Check sheet for the modelled part. Datum: model origin and axes. Units: mm. Face numbers are marked on the shaded views. A direction names the side the tool comes from. Coordinates: 2 decimals unless noted, no trailing zeros. Order: outer loops, then holes, each group sorted by start corner. A loop starts at its lowest first (then second) coordinate and runs counter-clockwise, first axis right, second up.
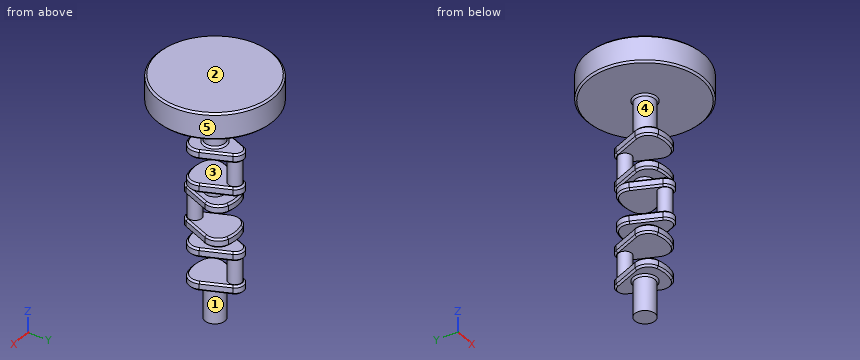
from build123d import *

# Parameters (mm, degrees)
SKETCH1_R             = 9.525
BOSS_EXTRUDE1_DEPTH   = 34.925
BOSS_EXTRUDE2_DEPTH   = 12.7
FILLET1_R             = 19.05
SKETCH3_R             = 14.2875
BOSS_EXTRUDE3_DEPTH   = 9.525
LPATTERN1_COUNT       = 3
LPATTERN1_PITCH       = 69.85
BODY_MOVE_COPY1_ANGLE = 180
LPATTERN2_COUNT       = 2
LPATTERN2_PITCH       = 69.85
SKETCH4_R             = 14.2875
BOSS_EXTRUDE4_DEPTH   = 57.15
BOSS_EXTRUDE5_START   = 50.8
SKETCH5_R             = 14.2875
BOSS_EXTRUDE5_DEPTH   = 50.8
SKETCH6_R             = 83.107085054
BOSS_EXTRUDE6_DEPTH   = 38.1
CHAMFER1_SIZE         = 2.54


with BuildPart() as part:
    # Sketch1 → Boss-Extrude1 (new body)
    with BuildSketch(Plane.XY):
        Circle(SKETCH1_R)
    extrude(amount=-BOSS_EXTRUDE1_DEPTH)

    # Sketch2 → Boss-Extrude2 (add)
    with BuildSketch(Plane(origin=(0, 0, -34.925), x_dir=(-1, 0, 0), z_dir=(0, 0, -1))):
        with BuildLine():
            Line((-11.733270063, 4.860079591), (-33.507418174, -47.707364088))
            ThreePointArc((-33.507418174, -47.707364088), (0, -60.325), (33.507418174, -47.707364088))
            Line((33.507418174, -47.707364088), (11.733270063, 4.860079591))
            ThreePointArc((11.733270063, 4.860079591), (0, 12.7), (-11.733270063, 4.860079591))
        make_face()
    extrude(amount=BOSS_EXTRUDE2_DEPTH)

    # Fillet1
    fillet1_edges = [part.edges().sort_by_distance(p)[0] for p in [
        (33.507418174, -47.707364088, -41.275),
        (-33.507418174, -47.707364088, -41.275),
    ]]
    fillet(fillet1_edges, radius=FILLET1_R)

    # Mirror2: part across plane


with BuildPart() as part_1:
    add(part.part)
    add(part.part.mirror(Plane.XY.offset(-17.4625)))


with BuildPart() as body_2:
    # Sketch3 → Boss-Extrude3 (new body)
    with BuildSketch(Plane(origin=(0, 0, -47.625), x_dir=(-1, 0, 0), z_dir=(0, 0, -1))):
        with Locations(Location((0, -28.486474017, 0), (0, 0, 180))):
            Circle(SKETCH3_R)
    boss_extrude3 = extrude(amount=BOSS_EXTRUDE3_DEPTH)


with BuildPart() as lpattern1_1:
    # LPattern1: pattern copy
    add(part_1.part.moved(Location(Vector(0, 0, -1) * (1 * LPATTERN1_PITCH))))


with BuildPart() as lpattern1_2:
    # LPattern1: pattern copy
    add(part_1.part.moved(Location(Vector(0, 0, -1) * (2 * LPATTERN1_PITCH))))

    # Sketch5 → Boss-Extrude5 (add)
    with BuildSketch(Plane(origin=(0, 0, -187.325), x_dir=(-1, 0, 0), z_dir=(0, 0, -1)).offset(BOSS_EXTRUDE5_START)):
        with Locations(Location((0, -28.486474017, 0), (0, 0, 180))):
            Circle(SKETCH5_R)
    extrude(amount=-BOSS_EXTRUDE5_DEPTH)


with BuildPart() as lpattern1_1_1:
    # Body-Move_Copy1: moved
    add(lpattern1_1.part.rotate(Axis((0, -28.486474017, 0), (0, 0, 1)), BODY_MOVE_COPY1_ANGLE))


with BuildPart() as lpattern2_1:
    # LPattern2: Boss-Extrude3 ×2
    with Locations(*[(0, 0, -i * LPATTERN2_PITCH) for i in range(1, LPATTERN2_COUNT)]):
        add(boss_extrude3)


with BuildPart() as part_2:
    add(part_1.part)

    # Sketch4 → Boss-Extrude4 (add)
    with BuildSketch(Plane.XY.offset(12.7)):
        with Locations((0, -28.486474017)):
            Circle(SKETCH4_R)
    extrude(amount=BOSS_EXTRUDE4_DEPTH)

    # Sketch6 → Boss-Extrude6 (add)
    with BuildSketch(Plane.XY.offset(69.85)):
        with Locations(Location((0, -28.486474017, 0), (0, 0, 180))):
            Circle(SKETCH6_R)
    extrude(amount=BOSS_EXTRUDE6_DEPTH)


with BuildPart() as body_2_1:
    add(body_2.part)

    # Combine1: union LPattern1_1, LPattern2_1, LPattern1_2, part
    add(lpattern1_1_1.part)
    add(lpattern2_1.part)
    add(lpattern1_2.part)
    add(part_2.part)

    # Chamfer1
    chamfer1_edges = [body_2_1.edges().sort_by_distance(p)[0] for p in [
        (0, -69.672948033, -104.775),
        (-19.470080331, -43.154715345, -104.775),
        (0, 3.352051967, -104.775),
        (19.470080331, -43.154715345, -104.775),
        (-19.470080331, -43.154715345, -117.475),
        (-26.88006293, -9.152399421, -117.475),
        (0, 3.352051967, -117.475),
        (26.88006293, -9.152399421, -117.475),
        (19.470080331, -43.154715345, -117.475),
        (0, -69.672948033, -117.475),
        (-26.88006293, -9.152399421, -104.775),
        (26.88006293, -9.152399421, -104.775),
        (0, -69.672948033, -57.15),
        (-19.470080331, -43.154715345, -57.15),
        (0, 3.352051967, -57.15),
        (19.470080331, -43.154715345, -57.15),
        (0, 3.352051967, -69.85),
        (19.470080331, -43.154715345, -69.85),
        (0, -69.672948033, -69.85),
        (-19.470080331, -43.154715345, -69.85),
        (-26.88006293, -9.152399421, -57.15),
        (-26.88006293, -9.152399421, -69.85),
        (26.88006293, -9.152399421, -57.15),
        (26.88006293, -9.152399421, -69.85),
        (0, 12.7, -174.625),
        (19.470080331, -13.818232688, -174.625),
        (0, -60.325, -174.625),
        (-19.470080331, -13.818232688, -174.625),
        (19.470080331, -13.818232688, -187.325),
        (26.88006293, -47.820548612, -187.325),
        (0, -60.325, -187.325),
        (-26.88006293, -47.820548612, -187.325),
        (-19.470080331, -13.818232688, -187.325),
        (0, 12.7, -187.325),
        (26.88006293, -47.820548612, -174.625),
        (-26.88006293, -47.820548612, -174.625),
        (0, 12.7, -127),
        (19.470080331, -13.818232688, -127),
        (0, -60.325, -127),
        (-19.470080331, -13.818232688, -127),
        (0, -60.325, -139.7),
        (-19.470080331, -13.818232688, -139.7),
        (0, 12.7, -139.7),
        (19.470080331, -13.818232688, -139.7),
        (26.88006293, -47.820548612, -127),
        (26.88006293, -47.820548612, -139.7),
        (-26.88006293, -47.820548612, -127),
        (-26.88006293, -47.820548612, -139.7),
        (-14.2875, -28.486474017, -187.325),
        (0, 12.7, -34.925),
        (19.470080331, -13.818232688, -34.925),
        (0, -60.325, -34.925),
        (-19.470080331, -13.818232688, -34.925),
        (19.470080331, -13.818232688, -47.625),
        (26.88006293, -47.820548612, -47.625),
        (0, -60.325, -47.625),
        (-26.88006293, -47.820548612, -47.625),
        (-19.470080331, -13.818232688, -47.625),
        (0, 12.7, -47.625),
        (26.88006293, -47.820548612, -34.925),
        (-26.88006293, -47.820548612, -34.925),
        (0, 12.7, 12.7),
        (19.470080331, -13.818232688, 12.7),
        (0, -60.325, 12.7),
        (-19.470080331, -13.818232688, 12.7),
        (0, -60.325, 0),
        (-19.470080331, -13.818232688, 0),
        (0, 12.7, 0),
        (19.470080331, -13.818232688, 0),
        (26.88006293, -47.820548612, 12.7),
        (26.88006293, -47.820548612, 0),
        (-26.88006293, -47.820548612, 12.7),
        (-26.88006293, -47.820548612, 0),
        (-14.2875, -28.486474017, 12.7),
        (83.107085054, -28.486474017, 69.85),
        (83.107085054, -28.486474017, 107.95),
        (-14.2875, -28.486474017, 69.85),
    ]]
    chamfer(chamfer1_edges, length=CHAMFER1_SIZE)


solid = body_2_1.part
(1) Cross-section at A-A (z = -18.5). Enter the section's corners in (x, y) (3 decimals), and give its area (3 significant figures).
Filled in:
outline: circle Ø19.05 at (0, 0)
area: 285 mm2
(2) Thickness scan on probe 1 along Z at (x, y) = (11.5, -22) (3 decimals); probe 2 along Z at (x, y) = (-30, -74); probe 3 along Z at (x, y) = (70, -68.5). Record the ranges inside material, lowest first.
Filled in:
probe 1: z = -238.125 to -174.625, -139.7 to -104.775, -69.85 to -34.925, 0 to 107.95
probe 2: z = 69.85 to 107.95
probe 3: z = 69.91 to 107.89
(3) Go/stop test with flat-tipped pins: P1, Ø12, axis at x = -17.5, z = -43.5, coming from the -Y side; P2, Ø1, axis at x = -27, y = 1.5, coming from the -Z side; P3, Ø8, axis at x = -14, z = -90, coming from the +Y side; P4, Ø4, axis at y = -2.5, z = -26.5, coming from the -X side. Record where each tip stops, or that it passes through.
Filled in:
P1: stops at y = -59.01
P2: stops at z = 69.85
P3: passes through
P4: stops at x = -9.51
(4) Release check for a two-part mould opening along Z. For the marked faces 1, 2 and 3 record: +Z half, -Z half, draft (parallel to the pull), parting line (faces both ways), or undercut.
Filled in:
face 1: draft
face 2: +Z half
face 3: undercut
(5) Tool access check on the marked faces 4 and 5. Record the directions out of +Z, -Z, +X, -X, +Y, -Y that give a thin tool (end or side, any length) a straight path to the whole face; none if there is none.
Filled in:
face 4: none
face 5: +Z, -Z
(6) Cross-section at B-B (z = -207.5). Enter the section's corners in (x, y) (1 decimal), and give its area (3 significant figures).
Filled in:
outline: circle Ø28.6 at (0, -28.5)
area: 641 mm2
